from build123d import *

# Parameters (mm, degrees)
SKETCH1_W           = 19
SKETCH1_H           = 20
SKETCH1_W_2         = 2
SKETCH1_H_2         = 5
BOSS_EXTRUDE1_DEPTH = 2
SKETCH2_W           = 5
SKETCH2_H           = 15
CUT_EXTRUDE1_DEPTH  = 10


with BuildPart() as part:
    # Sketch1 → Boss-Extrude1 (new body)
    with BuildSketch(Plane(origin=(0, 0, 0), x_dir=(1, 0, 0), z_dir=(0, 1, 0))):
        with Locations((5.5, 0)):
            Rectangle(SKETCH1_W, SKETCH1_H)
        with Locations((-1, 5)):
            Rectangle(SKETCH1_W_2, SKETCH1_H_2, mode=Mode.SUBTRACT)
        with Locations((-1, -5)):
            Rectangle(SKETCH1_W_2, SKETCH1_H_2, mode=Mode.SUBTRACT)
    extrude(amount=BOSS_EXTRUDE1_DEPTH)

    # Sketch2 → Cut-Extrude1 (cut)
    with BuildSketch(Plane(origin=(0, 2, 0), x_dir=(1, 0, 0), z_dir=(0, 1, 0))):
        with Locations((2.5, 0)):
            Rectangle(SKETCH2_W, SKETCH2_H)
    extrude(amount=-CUT_EXTRUDE1_DEPTH, mode=Mode.SUBTRACT)


solid = part.part
Can you work these out from the model? Positions are in its coordinate system, mm. A direction names the side the tool comes from. Coordinates: 2 decimals unless noted, no trailing zeros. Write each loop counter-clockwise with the first axis right and the second up, starting at its lowest first coordinate (ties: lowest second). Pieces come first, ordered by that corner, then holes. Notation, with made-up numbers: (49.5, 76.5) -> (89.5, 76.5) arc R29 cw to (89.5, 113.5) -> close; hole circle Ø10 at (6.25, -4). An arc over 180 degrees is marked (long way). Write each question's results on one line, items separated by ' | '. Start each with the question number.
Q1. Imagine slicing it at A-A (z = -0.25). Write out the boundary of the cut face in (x, y).
Q2. Imagine slicing it at D-D (z = 3). Write out the boundary of the cut face in (x, y).
Q3. If I drill on probe 1 along X at (y, z) = (0.6, 1.5); probe 2 along Z at (x, y) = (1.5, 0.45); probe 3 along X at (y, z) = (1.85, -3), over which ranges is the centre line in solid material (lowest first)?
Q4. We'd pull the mould along X, two halves only. Please class faces 3 (the face through (15, 1, 0)), 4 (the face through (7, 0, 0)), 5 (the face through (-2, 1, -5)): +X half, -X half, draft (parallel to the pull), parting line (faces both ways), or undercut.
Q5. Imagine slicing it at B-B (x = -0.5). Write out the boundary of the cut face in (y, z), then the cut area to 3 significant figures.
Q6. Imagine slicing it at C-C (y = 0.45). Write out the boundary of the cut face in (x, z).
Q7. On a 3-axis mill with a long thin cutter (end or side, diameter ignored), from which of +Z, -Z, +X, -X, +Y, -Y can I reach the whole of each face in a straight line? I mean faces 1 (the face through (5, 1, -10)), 2 (the face through (0, 1, 0)). Say none if no direction works.
Taken from the geometry:
1) outline: (-4, 0) -> (0, 0) -> (0, 2) -> (-4, 2) -> close; (5, 0) -> (15, 0) -> (15, 2) -> (5, 2) -> close
2) outline: (-4, 0) -> (-2, 0) -> (-2, 2) -> (-4, 2) -> close; (5, 0) -> (15, 0) -> (15, 2) -> (5, 2) -> close
3) probe 1: x = -4 to 0, 5 to 15 | probe 2: z = -10 to -7.5, 7.5 to 10 | probe 3: x = -4 to -2, 5 to 15
4) face 3: +X half | face 4: draft | face 5: undercut
5) outline: (0, -10) -> (2, -10) -> (2, -7.5) -> (0, -7.5) -> close; (0, -2.5) -> (2, -2.5) -> (2, 2.5) -> (0, 2.5) -> close; (0, 7.5) -> (2, 7.5) -> (2, 10) -> (0, 10) -> close | area: 20.0 mm^2
6) outline: (-4, -10) -> (15, -10) -> (15, 10) -> (-4, 10) -> close; hole (-2, -7.5) -> (5, -7.5) -> (5, 7.5) -> (-2, 7.5) -> (-2, 2.5) -> (0, 2.5) -> (0, -2.5) -> (-2, -2.5) -> close
7) face 1: -Z, +X, -X, +Y, -Y | face 2: +Y, -Y
